```python
from build123d import *

# Parameters (mm, degrees)
SKETCH1_W           = 20
SKETCH1_H           = 5
SKETCH1_W_2         = 5
SKETCH1_H_2         = 57
BOSS_EXTRUDE1_DEPTH = 30
FILLET1_R           = 4
SKETCH2_R           = 2
CUT_EXTRUDE1_DEPTH  = 30


with BuildPart() as part:
    # Sketch1 → Boss-Extrude1 (new body)
    with BuildSketch(Plane.XY):
        with Locations((-12.5, 26)):
            Rectangle(SKETCH1_W, SKETCH1_H)
        Rectangle(SKETCH1_W_2, SKETCH1_H_2)
        with Locations((12.5, -26)):
            Rectangle(SKETCH1_W, SKETCH1_H)
    extrude(amount=BOSS_EXTRUDE1_DEPTH)

    # Fillet1
    fillet1_edges = [part.edges().sort_by_distance(p)[0] for p in [
        (2.5, 28.5, 15),
        (2.5, -23.5, 15),
    ]]
    fillet(fillet1_edges, radius=FILLET1_R)

    # Sketch2 → Cut-Extrude1 (cut)
    with BuildSketch(Plane(origin=(0, -23.5, 0), x_dir=(1, 0, 0), z_dir=(0, 1, 0))):
        with Locations(Location((12.5, -15, 0), (0, 0, 270))):
            Circle(SKETCH2_R)
        with Locations(Location((12.5, -22.5, 0), (0, 0, 270))):
            Circle(SKETCH2_R)
        with Locations(Location((12.5, -7.5, 0), (0, 0, 270))):
            Circle(SKETCH2_R)
    extrude(amount=-CUT_EXTRUDE1_DEPTH, mode=Mode.SUBTRACT)


solid = part.part
```
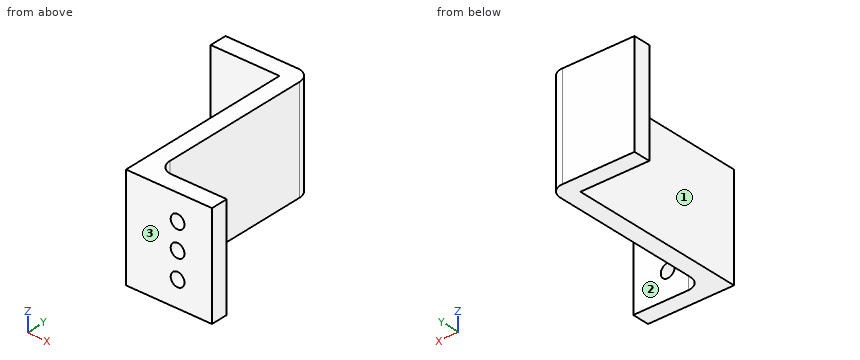
Could you check a few things on this model? Use its own coordinates, in mm. Face numbers are marked on the shaded views. A direction names the side the tool comes from. Give positions to 0.01 mm unless a question says otherwise; leave off trailing zeros. Order: outer loops, then holes, each group sorted by start corner. A loop starts at its lowest first (then second) coordinate and runs counter-clockwise, first axis right, second up.
Q1. For the marked faces 1, 2 and 3, which set-ups out of +Z, -Z, +X, -X, +Y, -Y let a thin tool reach every point of the face, with its end or its side?
Q2. Suppose I cut it at B-B, the plane z = 7.5. Write out the boundary of the cut face in (x, y), and give its area (3 significant figures).
Q3. Suppose I cut it at A-A, the plane x = 12.5. Write out the boundary of the cut face in (y, z), and give its area (3 significant figures).
Q4. I'm going to push flat-ended pins straight in: P1, Ø6, axis at x = 4.5, y = 9.5, coming from the +Z side; P2, Ø8, axis at y = 10.5, z = 8, coming from the -X side; P3, Ø4, axis at x = 11, z = 26, coming from the +Y side; P4, Ø6, axis at x = -10.5, z = 7.5, coming from the -Y side. Where does each tip first touch, or does it pass through?
Q5. Suppose I cut it at D-D, the plane y = -6.5. Write out the boundary of the cut face in (x, z).
Q6. Suppose I cut it at C-C, the plane z = 19.25. Write out the boundary of the cut face in (x, y), and give its area (3 significant figures).
Q7. If I drill on line 1 along Z through (x, y) = (12, -26); line 2 along X through (y, z) = (-26.55, 22.5); line 3 along Y through (x, z) = (-6.5, 22.25), over which ranges is the centre line in solid material (lowest first)?
Solution:
1. face 1: +Z, -Z, -X, -Y
1. face 2: +Z, -Z, +X, +Y
1. face 3: +Z, -Z, +X, -X, -Y
2. outline: (-22.5, 23.5) - (-2.5, 23.5) - (-2.5, -28.5) - (10.5, -28.5) - (10.5, -23.5) - (6.5, -23.5) arc R4 cw to (2.5, -19.5) - (2.5, 24.5) arc R4 ccw to (-1.5, 28.5) - (-22.5, 28.5) - close; (14.5, -28.5) - (22.5, -28.5) - (22.5, -23.5) - (14.5, -23.5) - close
2. area: 465 mm2
3. outline: (-28.5, 0) - (-23.5, 0) - (-23.5, 5.5) - (-28.5, 5.5) - close; (-28.5, 9.5) - (-23.5, 9.5) - (-23.5, 13) - (-28.5, 13) - close; (-28.5, 17) - (-23.5, 17) - (-23.5, 20.5) - (-28.5, 20.5) - close; (-28.5, 24.5) - (-23.5, 24.5) - (-23.5, 30) - (-28.5, 30) - close
3. area: 90.0 mm2
4. P1: stops at z = 30
4. P2: stops at x = -2.5
4. P3: stops at y = -23.5
4. P4: stops at y = 23.5
5. outline: (-2.5, 0) - (2.5, 0) - (2.5, 30) - (-2.5, 30) - close
6. outline: (-22.5, 23.5) - (-2.5, 23.5) - (-2.5, -28.5) - (22.5, -28.5) - (22.5, -23.5) - (6.5, -23.5) arc R4 cw to (2.5, -19.5) - (2.5, 24.5) arc R4 ccw to (-1.5, 28.5) - (-22.5, 28.5) - close
6. area: 485 mm2
7. line 1: z = 0 to 5.56, 9.44 to 13.06, 16.94 to 20.56, 24.44 to 30
7. line 2: x = -2.5 to 10.5, 14.5 to 22.5
7. line 3: y = 23.5 to 28.5
